Input: part model. Units: mm. Frame: model coordinates. Face numbers are marked on the shaded views. A direction names the side the tool comes from. Give positions to 0.01 mm unless a question says otherwise; leave off trailing zeros. Write each loop counter-clockwise with the first axis right and the second up, starting at its lowest first coordinate (ties: lowest second). Pieces come first, ordered by that corner, then holes. Notation, with made-up numbers: (57.25, 39.25) - (104.25, 39.25) arc R21 ccw to (104.25, 74.25) - close; hole circle Ø11 at (-7.75, 3). An arc over 180 degrees is marked (long way). Answer as CSV lines item,"result".
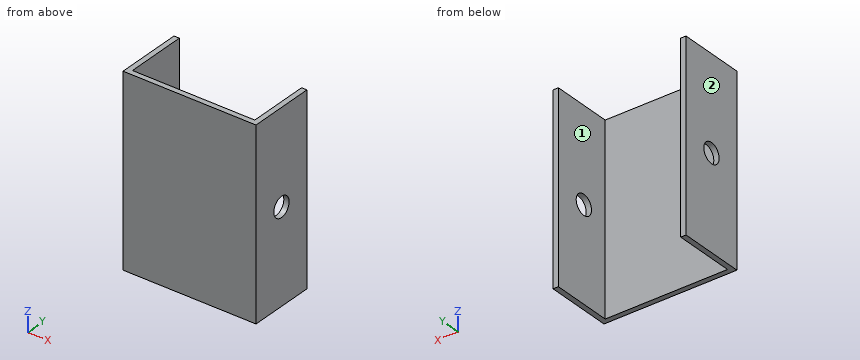
```python
from build123d import *

# Parameters (mm, degrees)
BOSS_EXTRUDE1_DEPTH     = 140
CUT_EXTRUDE1_DEPTH      = 174.980077517
CUT_EXTRUDE1_DEPTH_BACK = 174.980077517
SKETCH2_R               = 7.5


with BuildPart() as part:
    # Sketch1 → Boss-Extrude1 (new body)
    with BuildSketch(Plane.XY):
        Polygon((-38.824195441, 25.86633667), (-34.824195441, 25.86633667), (-34.824195441, -20.133663278), (57.175804455, -20.133663278), (57.175804455, 25.866336594), (61.175804559, 25.866336594), (61.175804559, -24.133663406), (-38.824195441, -24.133663406), align=None)
    extrude(amount=BOSS_EXTRUDE1_DEPTH)

    # Sketch2 → Cut-Extrude1 (cut, two sides: drawn at the far end of the back side and taken through both)
    with BuildSketch(Plane(origin=(61.175804559, 0, 0), x_dir=(0, 0, -1), z_dir=(1, 0, 0)).offset(-CUT_EXTRUDE1_DEPTH_BACK)):
        with Locations(Location((-70, 0.866336594, 0), (0, 0, 90))):
            Circle(SKETCH2_R)
    extrude(amount=CUT_EXTRUDE1_DEPTH + CUT_EXTRUDE1_DEPTH_BACK, mode=Mode.SUBTRACT)


solid = part.part
```
Item 1: Cut plane B-B on z = 70. Return the cut outline in (x, y).
The answers:
outline,"(-38.82, -24.13) - (61.18, -24.13) - (61.18, -6.63) - (57.18, -6.63) - (57.18, -20.13) - (-34.82, -20.13) - (-34.82, -6.63) - (-38.82, -6.63) - close; (-38.82, 8.37) - (-34.82, 8.37) - (-34.82, 25.87) - (-38.82, 25.87) - close; (57.18, 8.37) - (61.18, 8.37) - (61.18, 25.87) - (57.18, 25.87) - close"
Item 2: Cut plane D-D on z = 105.5. Return the cut outline in (x, y).
The answers:
outline,"(-38.82, -24.13) - (61.18, -24.13) - (61.18, 25.87) - (57.18, 25.87) - (57.18, -20.13) - (-34.82, -20.13) - (-34.82, 25.87) - (-38.82, 25.87) - close"
Item 3: Reachability of the marked faces 1 and 2 from +Z, -Z, +X, -X, +Y, -Y: full face, straight path, thin tool, end or side. Return the list, or none.
The answers:
face 1,"+Z, -Z, +Y"
face 2,"+Z, -Z, -X, +Y, -Y"
Item 4: Cut plane A-A on y = 10.5. Return the cut outline in (x, z), plus the area to 3 significant figures.
The answers:
outline,"(-38.82, 0) - (-34.82, 0) - (-34.82, 140) - (-38.82, 140) - close; (57.18, 0) - (61.18, 0) - (61.18, 140) - (57.18, 140) - close"
area,"1,120 mm²"
Item 5: Contact query for a flat-ended pin moving along its axis: pin 1 (8 mm diameter, centred on x = 16, z = 113.5, fed in from +Y). Output: stop coordinate, or through.
The answers:
pin 1,"y = -20.13"
Item 6: Cut plane C-C on y = -1.5. Return the cut outline in (x, z), plus the area to 3 significant figures.
The answers:
outline,"(-38.82, 0) - (-34.82, 0) - (-34.82, 62.88) - (-38.82, 62.88) - close; (-38.82, 77.12) - (-34.82, 77.12) - (-34.82, 140) - (-38.82, 140) - close; (57.18, 0) - (61.18, 0) - (61.18, 62.88) - (57.18, 62.88) - close; (57.18, 77.12) - (61.18, 77.12) - (61.18, 140) - (57.18, 140) - close"
area,"1,010 mm²"
Item 7: Ray query, line 1 (X direction, y = 16.5, z = 100); line 2 (Y direction, x = -36, z = 70); line 3 (Y direction, x = 8, z = 107). Return the intervals inside material, ascending. Write a range as from..to.
The answers:
line 1,"-38.82..-34.82, 57.18..61.18"
line 2,"-24.13..-6.63, 8.37..25.87"
line 3,"-24.13..-20.13"
